```python
from build123d import *

# Parameters (mm, degrees)
ESBO_O1_R                = 42.5
RESSALTO_EXTRUS_O1_DEPTH = 14
CORTE_EXTRUS_O1_START    = -3.2
CORTE_EXTRUS_O1_DEPTH    = 3.2
ESBO_O5_R                = 1.75
CORTE_EXTRUS_O2_DEPTH    = 62.066684862
PADR_OCIRCULAR1_COUNT    = 6
ESBO_O6_R                = 2.1
CORTE_EXTRUS_O3_DEPTH    = 5


with BuildPart() as part:
    # Esboço1 → Ressalto-extrusão1 (new body)
    with BuildSketch(Plane.XY):
        Circle(ESBO_O1_R)
    extrude(amount=RESSALTO_EXTRUS_O1_DEPTH)

    # Esboço3 → Corte-Revolução1 (revolve, cut)
    with BuildSketch(Plane(origin=(0, 0, 0), x_dir=(1, 0, 0), z_dir=(0, 1, 0))):
        Polygon((0, 0), (0, -14), (-9, -14), (-9, -12.6), (-12, -12.6), (-12, -12), (-13, -12), (-13, -7), (-36, -7), (-36, 0), align=None)
    revolve(axis=Axis((0, 0, 0), (0, 0, 1)), mode=Mode.SUBTRACT)

    # Esboço4 → Corte-extrusão1 (cut)
    with BuildSketch(Plane.XY.offset(14).offset(CORTE_EXTRUS_O1_START)):
        with BuildLine():
            Line((-3.75, 39.25), (-3.75, 42.334235555))
            ThreePointArc((-3.75, 42.334235555), (0, 42.5), (3.75, 42.334235555))
            Line((3.75, 42.334235555), (3.75, 39.25))
            ThreePointArc((3.75, 39.25), (0, 35.5), (-3.75, 39.25))
        make_face()
    corte_extrus_o1 = extrude(amount=CORTE_EXTRUS_O1_DEPTH, mode=Mode.SUBTRACT)

    # Esboço5 → Corte-extrusão2 (cut, through all)
    with BuildSketch(Plane.XY.offset(10.8)):
        with Locations((0, 39.25)):
            Circle(ESBO_O5_R)
    corte_extrus_o2 = extrude(amount=-CORTE_EXTRUS_O2_DEPTH, mode=Mode.SUBTRACT)

    # PadrãoCircular1: Corte-extrusão1, Corte-extrusão2 ×6 about axis
    padr_ocircular1_axis = Axis((0, 0, 0), (0, 0, 1))
    add([corte_extrus_o1.rotate(padr_ocircular1_axis, i * 360 / PADR_OCIRCULAR1_COUNT) for i in range(1, PADR_OCIRCULAR1_COUNT)], mode=Mode.SUBTRACT)
    add([corte_extrus_o2.rotate(padr_ocircular1_axis, i * 360 / PADR_OCIRCULAR1_COUNT) for i in range(1, PADR_OCIRCULAR1_COUNT)], mode=Mode.SUBTRACT)

    # Esboço6 → Corte-extrusão3 (cut)
    with BuildSketch(Plane.XY.offset(14)):
        with Locations((-17.5, 30)):
            Circle(ESBO_O6_R)
        with Locations((17.5, 30)):
            Circle(ESBO_O6_R)
        with Locations((17.5, -30)):
            Circle(ESBO_O6_R)
        with Locations((-17.5, -30)):
            Circle(ESBO_O6_R)
    extrude(amount=-CORTE_EXTRUS_O3_DEPTH, mode=Mode.SUBTRACT)


solid = part.part
```
CAD build for the part. Positions are in the model's coordinates, mm. A direction names the side the tool comes from. Give positions to 0.01 mm unless a question says otherwise; leave off trailing zeros. Loops run counter-clockwise (first coordinate to the right, second up) from the corner with the lowest first, then second, coordinate; pieces in that order, holes last. Notation, with made-up numbers: (80.5, 55.25) - (127.5, 55.25) arc R11 ccw to (127.5, 64.25) - close; hole circle Ø5 at (-7, 83.25). An arc over 180 degrees is marked (long way). Put each result on its own line as item: value.
Q1. Mould opens along Y. For faces 4 (the face through (-33.727, -25.861, 6.902)), 5 (the face through (-16.531, -31.863, 11.535)), 6 (the face through (37.22, 17.16, 12.38)), 7 (the face through (2, -9, 12.6)) say: pulls with the +Y half, pulls with the -Y half, needs draft (parallel to the pull), parting line crosses it, or undercut.
Filled in:
face 4: parting line crosses it
face 5: undercut
face 6: pulls with the +Y half
face 7: undercut
Q2. Slice it at B-B (x = 0). Give the number of separate pieces and of enclosed holes in the cut face, plus the area to 3 significant figures.
Filled in:
separate pieces: 4
enclosed holes: 0
area: 396 mm²
Q3. Tool access for faces 1 (the face through (30.786, 17.679, 12.378)), 2 (the face through (3.75, -41, 12)), 3 (the face through (0, 37, 10.8)): list every direction of +Z, -Z, +X, -X, +Y, -Y with a clear straight run to the whole face (end or side of a thin tool).
Filled in:
face 1: +Z
face 2: +Z, -Y
face 3: +Z, +Y
Q4. Probe line 1 along Y through (x, z) = (0, 9.15); line 2 along Y through (x, z) = (0, 12.25); line 3 along Y through (x, z) = (-32.5, 13). List the from-to ranges inside material, lowest first.
Filled in:
line 1: y = -42.5 to -41, -37.5 to -13, 13 to 37.5, 41 to 42.5
line 2: y = -35.5 to -12, 12 to 35.5
line 3: y = -27.39 to -23.09, -16.18 to 16.18, 23.09 to 27.39
Q5. Slice it at A-A (y = 0). Give the cut face in (x, z).
Filled in:
outline: (-42.5, 0) - (-36, 0) - (-36, 7) - (-13, 7) - (-13, 12) - (-12, 12) - (-12, 12.6) - (-9, 12.6) - (-9, 14) - (-42.5, 14) - close; (9, 12.6) - (12, 12.6) - (12, 12) - (13, 12) - (13, 7) - (36, 7) - (36, 0) - (42.5, 0) - (42.5, 14) - (9, 14) - close
Q6. Flat gauge pins, fed straight in: pin 1 (2 mm diameter, centred on x = 2, y = 38.5, fed in from +Z); pin 2 (2 mm diameter, centred on x = -17.5, y = 29, fed in from +Z); pin 3 (3 mm diameter, centred on x = 3, y = -17, fed in from -Z). Where does each tip first touch, or does it go through?
Filled in:
pin 1: stops at z = 10.8
pin 2: stops at z = 9
pin 3: stops at z = 7
Q7. Slice it at C-C (y = 20). Give the cut face in (x, z), plus the area to 3 significant figures.
Filled in:
outline: (-37.5, 0) - (-35.7, 0) - (-35.7, 10.8) - (-37.5, 10.8) - close; (-32.28, 0) - (-29.93, 0) - (-29.93, 7) - (29.93, 7) - (29.93, 0) - (32.28, 0) - (32.28, 10.8) - (30.26, 10.8) - (30.26, 14) - (-30.26, 14) - (-30.26, 10.8) - (-32.28, 10.8) - close; (35.7, 0) - (37.5, 0) - (37.5, 10.8) - (35.7, 10.8) - close
area: 511 mm²
